```python
from build123d import *

# Parameters (mm, degrees)
SKETCH1_R                = 12
MOTOR_HOUSING_DEPTH      = 31
SKETCH2_R                = 3
MOTOR_FRONT_NIPPLE_DEPTH = 1.5
SKETCH4_R                = 1
FRONT_AXLE_DEPTH         = 9
FILLET1_R                = 0.5
FILLET2_R                = 0.5
SKETCH5_R                = 4.5
BOSS_EXTRUDE1_DEPTH      = 2
BOSS_EXTRUDE2_START      = 1
SKETCH6_R                = 1
BOSS_EXTRUDE2_DEPTH      = 1
FILLET3_R                = 0.5


with BuildPart() as part:
    # Sketch1 → Motor housing (new body)
    with BuildSketch(Plane(origin=(0, 0, 0), x_dir=(1, 0, 0), z_dir=(0, 1, 0))):
        with Locations(Location((0, 0, 0), (0, 0, 270))):
            Circle(SKETCH1_R)
    extrude(amount=MOTOR_HOUSING_DEPTH)

    # Sketch2 → Motor front nipple (add)
    with BuildSketch(Plane(origin=(0, 31, 0), x_dir=(1, 0, 0), z_dir=(0, 1, 0))):
        with Locations(Location((0, 0, 0), (0, 0, 270))):
            Circle(SKETCH2_R)
    extrude(amount=MOTOR_FRONT_NIPPLE_DEPTH)

    # Sketch4 → Front axle (add)
    with BuildSketch(Plane(origin=(0, 32.5, 0), x_dir=(1, 0, 0), z_dir=(0, 1, 0))):
        with Locations(Location((0, 0, 0), (0, 0, 270))):
            Circle(SKETCH4_R)
    extrude(amount=FRONT_AXLE_DEPTH)

    # Fillet1
    fillet1_edges = [part.edges().sort_by_distance(p)[0] for p in [
        (0, 41.5, -1),
    ]]
    fillet(fillet1_edges, radius=FILLET1_R)

    # Fillet2
    fillet2_edges = [part.edges().sort_by_distance(p)[0] for p in [
        (0, 0, -12),
        (0, 31, -12),
    ]]
    fillet(fillet2_edges, radius=FILLET2_R)

    # Sketch5 → Boss-Extrude1 (add)
    with BuildSketch(Plane.XZ):
        with Locations(Location((0, 0, 0), (0, 0, 90))):
            Circle(SKETCH5_R)
    extrude(amount=BOSS_EXTRUDE1_DEPTH)

    # Sketch6 → Boss-Extrude2 (add)
    with BuildSketch(Plane.XZ.offset(2).offset(BOSS_EXTRUDE2_START)):
        with Locations(Location((0, 0, 0), (0, 0, 90))):
            Circle(SKETCH6_R)
    extrude(amount=-BOSS_EXTRUDE2_DEPTH)

    # Fillet3
    fillet3_edges = [part.edges().sort_by_distance(p)[0] for p in [
        (0, -2, -4.5),
        (0, -3, -1),
    ]]
    fillet(fillet3_edges, radius=FILLET3_R)


solid = part.part
```
Work out the finished part from the listing and answer in its coordinate system (mm). A direction names the side the tool comes from. Give positions to 0.01 mm unless a question says otherwise; leave off trailing zeros. Order: outer loops, then holes, each group sorted by start corner. A loop starts at its lowest first (then second) coordinate and runs counter-clockwise, first axis right, second up. Notation, with made-up numbers: (37, 43) -> (90, 43) arc R18 cw to (90, 63) -> close; hole circle Ø10 at (-36, -32). An arc over 180 degrees is marked (long way). Answer as CSV lines item,"result". Start each with the question number.
(1) Section A-A, the plane y = 13 is taken. Write down the section's boundary in (x, z).
(2) Consider line 1 along Y through (x, z) = (-5.5, 7.25); line 2 along X through (y, z) = (18.5, 0.5); line 3 along Y through (x, z) = (1.5, -0.5). Determine where each line is inside the solid, lowest interval first.
(3) Which of the six approach directions +Z, -Z, +X, -X, +Y, -Y give full straight-line access (tool end or side, diameter ignored) to faces 1 (the flat face through (0, -3, 0)), 2 (the flat face through (0, 0, 5)), 3 (the cylindrical face through (-1, 37, 0))?
(4) Section B-B, the plane y = 38 is taken. Write down the section's boundary in (x, z), plus the area to 3 significant figures.
(5) Each of these flat-tipped pins is pushed along its axis until it touches: pin 1 Ø5 at (x, z) = (1, -0.5) entering from +Y; pin 2 Ø6 at (x, z) = (3, -3.5) entering from +Y; pin 3 Ø3 at (x, y) = (-3.5, 23.5) entering from -Z; pin 4 Ø7 at (x, z) = (-4.5, -4.5) entering from -Y. Where does it stop, or does it pass through?
Entries:
1,outline,"circle Ø24 at (0, 0)"
2,line 1,"0 to 31"
2,line 2,"-11.99 to 11.99"
2,line 3,"-2 to 32.5"
3,face 1,"+Z, -Z, +X, -X, -Y"
3,face 2,"-Y"
3,face 3,"+Y"
4,outline,"circle Ø2 at (0, 0)"
4,area,"3.14 mm²"
5,pin 1,"y = 41.5"
5,pin 2,"y = 32.5"
5,pin 3,"z = -11.83"
5,pin 4,"y = -2"
